```python
from build123d import *

# Parameters (mm, degrees)
SKETCH_R     = 21
PAD_DEPTH    = 15
SKETCH001_W  = 10
SKETCH001_H  = 10
POCKET_DEPTH = 5
SKETCH002_R  = 8
PAD001_DEPTH = 30


with BuildPart() as part:
    # Sketch → Pad (new body)
    with BuildSketch(Plane.XZ):
        Circle(SKETCH_R)
    extrude(amount=PAD_DEPTH)

    # Sketch001 → Pocket (cut)
    with BuildSketch(Plane.XZ.offset(15)):
        Rectangle(SKETCH001_W, SKETCH001_H)
    extrude(amount=-POCKET_DEPTH, mode=Mode.SUBTRACT)

    # Sketch002 → Pad001 (new body)
    with BuildSketch(Plane(origin=(0, 0, 0), x_dir=(1, 0, 0), z_dir=(0, 1, 0))):
        Circle(SKETCH002_R)
    extrude(amount=PAD001_DEPTH)


solid = part.part
```
Geometry check sheet. Reference: the model listing, model coordinates, mm. A direction names the side the tool comes from. Coordinates: 2 decimals unless noted, no trailing zeros. Order: outer loops, then holes, each group sorted by start corner. A loop starts at its lowest first (then second) coordinate and runs counter-clockwise, first axis right, second up. Notation, with made-up numbers: M -26.5,89 L 13.5,89 A17 cw 13.5,105 Z; hole C 47,-38.75 d6. An arc over 180 degrees is marked long. Answer as a JSON object with one key per item and string values.
Q1. Scan lines: line 1 (Y direction, x = 3, z = 3.5); line 2 (Y direction, x = -0.5, z = -18); line 3 (X direction, y = -6, z = -5). Record each from-to range of solid material in increasing order.
Results are:
{"line 1": "y = -10 to 30", "line 2": "y = -15 to 0", "line 3": "x = -20.4 to 20.4"}
Q2. Cross-section at D-D on z = 15.5. Record the cut outline in (x, y).
Results are:
{"outline": "M -14.17,-15 L 14.17,-15 L 14.17,0 L -14.17,0 Z"}
Q3. Tool access check on faces 1 (the flat face through (0, 30, 0)), 2 (the flat face through (0, -13, -5)), 3 (the flat face through (9, 0, 0)). Record the directions out of +Z, -Z, +X, -X, +Y, -Y that give a thin tool (end or side, any length) a straight path to the whole face; none if there is none.
Results are:
{"face 1": "+Z, -Z, +X, -X, +Y", "face 2": "-Y", "face 3": "+Y"}
Q4. Cross-section at C-C on y = 17.5. Record the cut outline in (x, z).
Results are:
{"outline": "C 0,0 d16"}
Q5. Cross-section at B-B on z = 0. Record the cut outline in (x, y), and give its area (3 significant figures).
Results are:
{"outline": "M -21,-15 L -5,-15 L -5,-10 L 5,-10 L 5,-15 L 21,-15 L 21,0 L 8,0 L 8,30 L -8,30 L -8,0 L -21,0 Z", "area": "1,060 mm²"}
Q6. Depth check by flat-ended pin: pin 1 Ø6 at (x, y) = (8, -6) entering from +Z; pin 2 Ø3 at (x, z) = (-13.5, 16) entering from +Y; pin 3 Ø1.5 at (x, y) = (-1.5, -13.5) entering from -Z. Enter the tip coordinate at first touch or a pass-through.
Results are:
{"pin 1": "stops at z = 20.4", "pin 2": "stops at y = 0", "pin 3": "stops at z = -20.99"}
Q7. Release check for a two-part mould opening along Z. For faces 4 (the cylindrical face through (20.03, -7.4, 6.31)), 5 (the flat face through (9, -15, 0)), 6 (the flat face through (0, -10, 0)) record: released by +Z, released by -Z, zero draft, split by the parting line, or undercut.
Results are:
{"face 4": "split by the parting line", "face 5": "zero draft", "face 6": "undercut"}
Q8. Cross-section at A-A on x = 0. Record the cut outline in (y, z), and give its area (3 significant figures).
Results are:
{"outline": "M -15,-21 L 0,-21 L 0,-8 L 30,-8 L 30,8 L 0,8 L 0,21 L -15,21 L -15,5 L -10,5 L -10,-5 L -15,-5 Z", "area": "1,060 mm²"}
